```python
from build123d import *

# Parameters (mm, degrees)
SKETCH1_W           = 60
SKETCH1_H           = 120
BOSS_EXTRUDE1_DEPTH = 55
CUT_EXTRUDE1_DEPTH  = 146
SKETCH3_W           = 30
SKETCH3_H           = 30
CUT_EXTRUDE2_DEPTH  = 136.369863707
SKETCH5_R           = 7.5
CUT_EXTRUDE3_DEPTH  = 136.369863707
SKETCH6_R           = 7.5
CUT_EXTRUDE4_DEPTH  = 128.279220614


with BuildPart() as part:
    # Sketch1 → Boss-Extrude1 (new body)
    with BuildSketch(Plane(origin=(0, 0, 0), x_dir=(1, 0, 0), z_dir=(0, 1, 0))):
        with Locations((0, 60)):
            Rectangle(SKETCH1_W, SKETCH1_H)
    extrude(amount=BOSS_EXTRUDE1_DEPTH)

    # Sketch2 → Cut-Extrude1 (cut, through all)
    with BuildSketch(Plane(origin=(30, 0, 0), x_dir=(0, 0, -1), z_dir=(1, 0, 0))):
        Polygon((0, 0), (60, 55), (0, 55), align=None)
    extrude(amount=-CUT_EXTRUDE1_DEPTH, mode=Mode.SUBTRACT)

    # Sketch3 → Cut-Extrude2 (cut, through all)
    with BuildSketch(Plane(origin=(0, 0, -120), x_dir=(-1, 0, 0), z_dir=(0, 0, -1))):
        with Locations((-15, 40)):
            Rectangle(SKETCH3_W, SKETCH3_H)
    extrude(amount=-CUT_EXTRUDE2_DEPTH, mode=Mode.SUBTRACT)

    # Sketch5 → Cut-Extrude3 (cut, through all)
    with BuildSketch(Plane(origin=(0, 0, 0), x_dir=(0, 0, -1), z_dir=(1, 0, 0))):
        with Locations((100, 40)):
            Circle(SKETCH5_R)
    extrude(amount=-CUT_EXTRUDE3_DEPTH, mode=Mode.SUBTRACT)

    # Sketch6 → Cut-Extrude4 (cut, through all)
    with BuildSketch(Plane(origin=(0, 25, 0), x_dir=(1, 0, 0), z_dir=(0, 1, 0))):
        with Locations(Location((15, 60, 0), (0, 0, 270))):
            Circle(SKETCH6_R)
    extrude(amount=-CUT_EXTRUDE4_DEPTH, mode=Mode.SUBTRACT)


solid = part.part
```
Input: part model. Units: mm. Frame: model coordinates. A direction names the side the tool comes from. Coordinates: 2 decimals unless noted, no trailing zeros. Loops run counter-clockwise (first coordinate to the right, second up) from the corner with the lowest first, then second, coordinate; pieces in that order, holes last. Notation, with made-up numbers: M 41,20 L 56,20 A20 ccw 56,57 Z; hole C -3,58 d10. An arc over 180 degrees is marked long. Use a Markdown table: item, result. Add a question column.
1) Section C-C, the plane x = -8. Return the cut outline in (y, z), plus the area to 3 significant figures.
2) Section B-B, the plane y = 34. Return the cut outline in (x, z), plus the area to 3 significant figures.
3) Pin query (flat end, axial travel): P1, Ø5, axis at x = 9, z = -40, coming from the +Y side; P2, Ø2, axis at x = -23, z = -26.5, coming from the -Y side; P3, Ø3, axis at x = 17, y = 12, coming from the +Z side; P4, Ø10, axis at x = -20, y = 30, coming from the +Z side. Return the tip coordinate at first contact, or that it passes through.
4) Section D-D, the plane z = -30. Return the cut outline in (x, y), plus the area to 4 significant figures.
5) Set-up query: faces 5 (the flat face through (-30, 21, -72)), 6 (the flat face through (15, 25, -74)). Return all of +Z, -Z, +X, -X, +Y, -Y with unobstructed straight access to the full face (end or side cutting, diameter ignored); none if empty.
6) Line query: L1, parallel to Y at x = -17.25, z = -100; L2, parallel to X at y = 15, z = -60; L3, parallel to Y at x = 1.5, z = -79. Output: solid intervals per line, ascending. Write a range as from..to.
7) Section A-A, the plane x = 15. Return the cut outline in (y, z), plus the area to 3 significant figures.
8) Draft query along Y for faces 1 (the flat face through (-6.25, 21, -22.91)), 2 (the cylindrical face through (-14.79, 32.68, -98.37)), 3 (the flat face through (0, 0, -61)), 4 (the flat face through (-7, 21, -120)). Return one class per face: +Y half, -Y half, draft (parallel to the pull), parting line (faces both ways), or undercut.
Answer below:
| question | item | result |
|---|---|---|
| 1 | outline | M 0,-120 L 55,-120 L 55,-60 L 0,0 Z; hole C 40,-100 d15 |
| 1 | area | 4,770 mm2 |
| 2 | outline | M -30,-120 L 0,-120 L 0,-104.5 L -30,-104.5 Z; M -30,-95.5 L 0,-95.5 L 0,-37.09 L -30,-37.09 Z |
| 2 | area | 2,220 mm2 |
| 3 | P1 | y = 25 |
| 3 | P2 | y = 0 |
| 3 | P3 | z = -11.45 |
| 3 | P4 | z = -27.27 |
| 4 | outline | M -30,0 L 30,0 L 30,25 L 0,25 L 0,27.5 L -30,27.5 Z |
| 4 | area | 1,575 mm2 |
| 5 | face 5 | +Z, -Z, -X, +Y, -Y |
| 5 | face 6 | +Z, -Z, +X, +Y |
| 6 | L1 | 0..32.5, 47.5..55 |
| 6 | L2 | -30..7.5, 22.5..30 |
| 6 | L3 | 0..25 |
| 7 | outline | M 0,-120 L 25,-120 L 25,-67.5 L 0,-67.5 Z; M 0,-52.5 L 25,-52.5 L 25,-27.27 L 0,0 Z |
| 7 | area | 2,280 mm2 |
| 8 | face 1 | +Y half |
| 8 | face 2 | undercut |
| 8 | face 3 | -Y half |
| 8 | face 4 | draft |
